Design review of the part built by this model. Coordinates are the model's own, in mm. Face numbers are marked on the shaded views. A direction names the side the tool comes from. Round coordinates to 2 decimals unless told otherwise and drop trailing zeros. Order: outer loops, then holes, each group sorted by start corner. A loop starts at its lowest first (then second) coordinate and runs counter-clockwise, first axis right, second up. Notation, with made-up numbers: (53.5, -28.75) - (85.5, -28.75) arc R4 cw to (85.5, -21.75) - close; hole circle Ø6 at (-2.75, 65.25). An arc over 180 degrees is marked (long way). Use CSV: the item, a comma, the result in double quotes.
Autodesk Inventor part; units mm, degrees
ref_plane "YZ Plane" through (0, 0, 0) normal (1, 0, 0) x (0, 1, 0)
ref_plane "XZ Plane" through (0, 0, 0) normal (0, 1, 0) x (-1, 0, 0)
ref_plane "XY Plane" through (0, 0, 0) normal (0, 0, 1) x (1, 0, 0)
sketch "Sketch1" plane through (0, 0, 0) normal (0, 1, 0) x (-1, 0, 0)
  line L0 (-7.5, 5.5) -> (7.5, 5.5)
  line L1 (7.5, 5.5) -> (7.5, -5.5)
  line L2 (7.5, -5.5) -> (-7.5, -5.5)
  line L3 (-7.5, -5.5) -> (-7.5, 5.5)
  line L4 (-7.5, 5.5) -> (7.5, -5.5) construction
  line L5 (7.5, 5.5) -> (-7.5, -5.5) construction
  circle A0 centre (0, -5.5) radius 7.5 construction
  arc A1 (-7.5, -5.5) -> (7.5, -5.5) centre (0, -5.5) ccw
  point P0 (0, 0)
  dimension "d0" = 11
  dimension "d1" = 15
extrude "Extrusion1" add sketch "Sketch1" along normal blind 8
sketch "Sketch2" plane through (0, 0, 0) normal (0, -1, 0) x (1, 0, 0)
  line L0 (7.5, 9.25) -> (-7.5, 9.25)
  line L1 (-7.5, 9.25) -> (-7.5, -20.75)
  line L2 (-7.5, -20.75) -> (7.5, -20.75)
  line L3 (7.5, -20.75) -> (7.5, 9.25)
  line L4 (7.5, 9.25) -> (-7.5, -20.75) construction
  line L5 (-7.5, 9.25) -> (7.5, -20.75) construction
  line L6 (-7.5, 5.5) -> (7.5, 5.5)
  line L7 (7, 8.75) -> (-7, 8.75) construction
  line L8 (-7, 8.75) -> (-7, -20.25) construction
  line L9 (-7, -20.25) -> (7, -20.25) construction
  line L10 (7, -20.25) -> (7, 8.75) construction
  line L11 (7, 8.75) -> (-7, -20.25) construction
  line L12 (-7, 8.75) -> (7, -20.25) construction
  point P0 (0, 0)
  point P1 (0, -5.75)
  dimension "d4" = 15
  dimension "d5" = 30
  dimension "d6" = 3.75
  dimension "d18" = 0.5
  dimension "d19" = 0.5
sketch "Sketch4" plane through (0, 0, 0) normal (0, -1, 0) x (1, 0, 0)
  line L0 (-7.5, -5.5) -> (-7.5, 5.5)
  line L1 (-7.5, 3.75) -> (-6.5, 3.75)
  line L2 (-6.5, 3.75) -> (-6.5, 0.75)
  line L3 (-6.5, 0.75) -> (-7.5, 0.75)
  line L4 (-7.5, 0.75) -> (-7.5, 3.75)
  line L5 (7.5, 5.5) -> (7.5, -5.5)
  line L6 (7.5, 0.75) -> (6.5, 0.75)
  line L7 (6.5, 0.75) -> (6.5, 3.75)
  line L8 (6.5, 3.75) -> (7.5, 3.75)
  line L9 (7.5, 3.75) -> (7.5, 0.75)
  line L10 (-7.5, -20.25) -> (7.5, -20.25) construction
  line L11 (7.5, -20.25) -> (7.5, 9.75) construction
  line L12 (7.5, 9.75) -> (-7.5, 9.75) construction
  line L13 (-7.5, 9.75) -> (-7.5, -20.25) construction
  line L14 (-7.5, -20.25) -> (7.5, 9.75) construction
  line L15 (7.5, -20.25) -> (-7.5, 9.75) construction
  line L16 (-7.5, 5.5) -> (7.5, 5.5) construction
  arc A0 (-7.5, -5.5) -> (7.5, -5.5) centre (0, -5.5) ccw construction
  point P0 (0, 0)
  point P1 (0, -5.25)
  point P2 (0, -13)
  point P3 (-7, 3.75)
  point P4 (-7.5, 0.75)
  point P5 (-7, 0.75)
  point P6 (7.5, 3.75)
  point P7 (-7.5, 0.75)
  dimension "d20" = 1
  dimension "d21" = 3
  dimension "d22" = 1
  dimension "d23" = 3
  dimension "d24" = 15
  dimension "d25" = 30
  dimension "d27" = 7.25
  dimension "d106" = 0.75
extrude "Extrusion3" add sketch "Sketch4" along normal blind 1.6
sketch "Sketch6" plane through (0, 0, 0) normal (0, -1, 0) x (1, 0, 0)
  line L0 (7.5, 11.25) -> (-7.5, 11.25)
  line L1 (-7.5, 11.25) -> (-7.5, -18.75)
  line L2 (-7.5, -18.75) -> (7.5, -18.75)
  line L3 (7.5, -18.75) -> (7.5, 11.25)
  line L4 (7.5, 11.25) -> (-7.5, -18.75) construction
  line L5 (-7.5, 11.25) -> (7.5, -18.75) construction
  line L6 (7, 10.75) -> (-7, 10.75) construction
  line L7 (-7, 10.75) -> (-7, -18.25) construction
  line L8 (-7, -18.25) -> (7, -18.25) construction
  line L9 (7, -18.25) -> (7, 10.75) construction
  line L10 (7, 10.75) -> (-7, -18.25) construction
  line L11 (-7, 10.75) -> (7, -18.25) construction
  circle A0 centre (0, -3.75) radius 1
  circle A1 centre (0, -3.75) radius 1.5
  line L12 (-6.5, 4.5) -> (6.5, 4.5)
  line L13 (6.5, 4.5) -> (6.5, -5.5)
  line L14 (6.5, -5.5) -> (-6.5, -5.5)
  line L15 (-6.5, -5.5) -> (-6.5, 4.5)
  line L16 (-7.5, 5.5) -> (7.5, 5.5)
  arc A2 (-7.5, -5.5) -> (7.5, -5.5) centre (0, -5.5) ccw
  circle A3 centre (0, -5.5) radius 6.5
  point P0 (0, 0)
  point P1 (-7.5, -3.75)
  point P2 (6.5, -5.5)
  dimension "d31" = 15
  dimension "d32" = 30
  dimension "d34" = 0.5
  dimension "d35" = 0.5
  dimension "d36" = 2
  dimension "d37" = 0.5
  dimension "d38" = 1
  dimension "d39" = 1
  dimension "d40" = 1
  dimension "d41" = 1
  dimension "d107" = 3.75
extrude "Extrusion4" cut sketch "Sketch6" against normal blind 2.5 contours A0 | L12 L13 A3 L15 | A3 L14 | L14 A3
sketch "Sketch10" plane through (0, 8, 0) normal (0, 1, 0) x (1, 0, 0)
  point P0 (0, 0)
sketch "Sketch11" plane through (0, 0, 0) normal (0, -1, 0) x (1, 0, 0)
  line L0 (-5, 3.5) -> (-2.5, 3.5)
  line L1 (-2.5, 3.5) -> (-2.5, 2)
  line L2 (-2.5, 2) -> (-5, 2)
  line L3 (-5, 2) -> (-5, 3.5)
  line L4 (2.5, 3.5) -> (5, 3.5)
  line L5 (5, 3.5) -> (5, 2)
  line L6 (5, 2) -> (2.5, 2)
  line L7 (2.5, 2) -> (2.5, 3.5)
  line L8 (-6.5, 3.75) -> (-7.5, 3.75)
  line L9 (-6.5, 0.75) -> (-6.5, 3.75)
  line L10 (6.5, 3.75) -> (6.5, 0.75)
  line L11 (-6.5, 4.5) -> (6.5, 4.5)
  line L12 (-1.25, -11) -> (1.25, -11)
  line L13 (1.25, -11) -> (1.25, -9.5)
  line L14 (1.25, -9.5) -> (-1.25, -9.5)
  line L15 (-1.25, -9.5) -> (-1.25, -11)
  circle A0 centre (0, -3.75) radius 1
  point P0 (0, 0)
  point P1 (-3.75, 3.5)
  point P2 (3.75, 3.5)
  point P3 (1.25, -10.25)
  point P4 (2.5, 2.75)
  point P5 (0, -9.5)
  point P6 (3.75, 2)
  point P7 (-2.5, 2.75)
  dimension "d51" = 2.5
  dimension "d52" = 1.5
  dimension "d55" = 2.75
  dimension "d56" = 2.75
  dimension "d60" = 13
  dimension "d61" = 3.75
  dimension "d62" = 3.75
  dimension "d103" = 6.5
  dimension "d104" = 6.5
extrude "Extrusion8" cut sketch "Sketch11" against normal blind 10 contours L0 L1 L2 L3 | L4 L5 L6 L7 | L15 L14 L13 L12
sketch "Sketch12" plane through (0, 2.5, 0) normal (0, -1, 0) x (1, 0, 0)
  line L0 (5, 2) -> (5, 3.5) construction
  line L1 (2.5, 2) -> (5, 2) construction
  line L2 (5, 3.5) -> (2.5, 3.5) construction
  line L3 (2.5, 3.5) -> (2.5, 2) construction
  line L4 (2.5, 2) -> (5, 2) construction
  line L5 (5, 2) -> (5, 3.5) construction
  line L6 (-2.5, 2) -> (-2.5, 3.5) construction
  line L7 (-2.5, 2) -> (-5, 2) construction
  line L8 (-2.5, 3.5) -> (-5, 3.5) construction
  line L9 (-5, 3.5) -> (-5, 2) construction
  line L10 (-5, 2) -> (-2.5, 2) construction
  line L11 (-2.5, 2) -> (-2.5, 3.5) construction
  line L12 (-1.25, -9.5) -> (1.25, -9.5) construction
  line L13 (-1.25, -9.5) -> (-1.25, -11) construction
  line L14 (1.25, -9.5) -> (-1.25, -9.5) construction
  line L15 (-1.25, -9.5) -> (-1.25, -11) construction
  line L16 (-1.25, -11) -> (1.25, -11) construction
  line L17 (1.25, -11) -> (1.25, -9.5) construction
  line L18 (5.5, 3.5) -> (2, 3.5)
  line L19 (2, 3.5) -> (2, 2)
  line L20 (2, 2) -> (5.5, 2)
  line L21 (5.5, 2) -> (5.5, 3.5)
  line L22 (1.75, -9.5) -> (-1.75, -9.5)
  line L23 (-1.75, -9.5) -> (-1.75, -11)
  line L24 (-1.75, -11) -> (1.75, -11)
  line L25 (1.75, -11) -> (1.75, -9.5)
  line L26 (-2, 3.5) -> (-5.5, 3.5)
  line L27 (-5.5, 3.5) -> (-5.5, 2)
  line L28 (-5.5, 2) -> (-2, 2)
  line L29 (-2, 2) -> (-2, 3.5)
  point P0 (0, 0)
  point P1 (-2.5, 2.75)
  point P2 (-2, 2.75)
  point P3 (-3.75, 2)
  point P4 (-3.75, 2)
  point P5 (-3.75, 3.5)
  point P6 (-3.75, 3.5)
  point P7 (-5, 2.75)
  point P8 (-5.5, 2.75)
  point P9 (1.25, -10.25)
  point P10 (1.75, -10.25)
  point P11 (0, -11)
  point P12 (-1.25, -10.25)
  dimension "d63" = 0.5
  dimension "d64" = 0
  dimension "d65" = 0
  dimension "d67" = 0.5
  dimension "d68" = 0
  dimension "d69" = 0
  dimension "d70" = 0.5
  dimension "d71" = 0.5
  dimension "d72" = 0
  dimension "d73" = 0
  dimension "d74" = 0.5
  dimension "d96" = 0.5
extrude "Extrusion9" cut sketch "Sketch12" against normal blind 1
sketch "Sketch16" plane through (0, 2.5, 0) normal (0, -1, 0) x (1, 0, 0)
  line L0 (-6.5, -5.5) -> (-6.5, 4.5) construction
  line L1 (-6.5, 4.5) -> (6.5, 4.5) construction
  line L2 (-6.5, 4.5) -> (6.5, 4.5) construction
  line L3 (-0.5, 4.5) -> (0.5, 4.5)
  line L4 (0.5, 4.5) -> (0.5, -2.75)
  line L5 (0.5, -2.75) -> (-0.5, -2.75)
  line L6 (-0.5, -2.75) -> (-0.5, 4.5)
  circle A0 centre (0, -3.75) radius 1.5 construction
  circle A1 centre (0, -3.75) radius 1.75 construction
  line L7 (-6.5, -2.75) -> (6.5174, -2.75) construction
  circle A2 centre (0, -3.75) radius 1.5 construction
  circle A3 centre (0, -3.75) radius 1 construction
  line L8 (6.5, 0.75) -> (6.5, -5.5)
  line L9 (-6.5, -5.873) -> (6.5, -5.873)
  line L10 (6.5, -5.873) -> (6.5, -6.873)
  line L11 (6.5, -6.873) -> (-6.5, -6.873)
  line L12 (-6.5, -6.873) -> (-6.5, -5.873)
  point P0 (0, 0)
  point P1 (0, 4.5)
  point P2 (0.0087, -2.75)
  dimension "d94" = 1
  dimension "d95" = 1
extrude "Extrusion10" add sketch "Sketch16" along normal blind 2.5 contours L3 L4 L5 L6
sketch "Sketch19" plane through (-7.5, 0, 5.5) normal (0, 0, 1) x (1, 0, 0)
  line L0 (15, 0) -> (15, 8)
  line L1 (0, 8) -> (15, 8)
  line L2 (15, 8) -> (15, 0)
  line L3 (15, 0) -> (0, 0)
  line L4 (0, 0) -> (0, 8)
  point P0 (7.5, 0)
extrude "Extrusion13" add sketch "Sketch19" along normal blind 6
sketch "Sketch18" plane through (0, 8, 0) normal (0, 1, 0) x (1, 0, 0)
  line L0 (-7.5, -3.75) -> (-7.5, -5.5)
  line L1 (-7.5, -5.5) -> (-7.5, -8.2917)
  line L2 (7.5, -5.5) -> (7.5, -8.2917)
  arc A0 (7.5, -8.2917) -> (-7.5, -8.2917) centre (0, -17.6592) ccw
  line L3 (-7.5, -5.5) -> (0, -3.75)
  line L4 (-7.5, -5.5) -> (7.5, -5.5)
  line L5 (0, -3.75) -> (7.5, -5.5)
  line L6 (-7.5, -8.2917) -> (-7.5, -17.8663)
  line L7 (-7.5, -17.8663) -> (8.2387, -17.8663)
  line L8 (8.2387, -17.8663) -> (7.5, -8.2917)
  line L9 (-7.5, -8.2917) -> (-7.5, -5.5)
  point P0 (0, 0)
  point P1 (3.395, -5.5)
  point P2 (-3.395, -5.5)
  dimension "d108" = 12
extrude "Extrusion12" cut sketch "Sketch18" against normal blind 8 contours A0 L8 L7 L6
sketch "Sketch21" plane through (0, 8, 0) normal (0, 1, 0) x (1, 0, 0)
  line L0 (-7.5, 5.5) -> (-7.5, -8.2917)
  line L1 (-7.5, 5.5) -> (-4.5586, 5.5)
  line L2 (-4.5586, 5.5) -> (-4.5586, 13.4633)
  line L3 (-4.5586, 13.4633) -> (-7.5, 13.4633)
  line L4 (-7.5, 13.4633) -> (-7.5, 5.5)
  arc A0 (7.5, 5.5) -> (-7.5, 5.5) centre (0, 5.5) ccw
  line L5 (7.5, 5.5) -> (3.8632, 5.5)
  line L6 (3.8632, 5.5) -> (3.8632, 13.1156)
  line L7 (3.8632, 13.1156) -> (7.5, 13.1156)
  line L8 (7.5, 13.1156) -> (7.5, 5.5)
  point P0 (0, 0)
  point P1 (3.8632, 11.9285)
  point P2 (-4.5586, 11.4556)
  point P3 (-7.5, -5.5)
extrude "Extrusion15" add sketch "Sketch21" against normal blind 8 contours L6 L7 L8 A0 | L4 L3 L2 A0
sketch "Sketch20" plane through (0, 8, 0) normal (0, 1, 0) x (1, 0, 0)
  arc A0 (7.5, 5.5) -> (-7.5, 5.5) centre (0, 5.5) ccw
  line L0 (-7.5, 5.5) -> (-7.5, 7.5)
  line L1 (7.5, 5.5) -> (7.5, 7.5)
  arc A1 (0, 13) -> (-7.5, 7.5) centre (1.4853, 3.1109) ccw
  arc A2 (7.5, 7.5) -> (0, 13) centre (-1.4853, 3.1109) ccw
  line L2 (-7.5, 7.5) -> (-7.5, 19.3065)
  line L3 (-7.5, 7.5) -> (4.3065, 7.5) construction
  line L4 (-7.5, 19.3065) -> (7.5, 19.3065)
  line L5 (7.5, 19.3065) -> (7.5, 7.5)
  point P0 (0, 0)
  point P1 (-6.7259, 8.8184)
  point P2 (6.7259, 8.8184)
  dimension "d113" = 2
  dimension "d114" = 10
  dimension "d115" = 90
  dimension "d116" = 90
extrude "Extrusion14" cut sketch "Sketch20" against normal blind 10 contours A2 A0 | A0 A1 L2 L4 L5 A2 | A1 A0
sketch "Sketch23" plane through (0, 2.5, -3.75) normal (0, -1, 0) x (1, 0, 0)
  circle A0 centre (0, 0) radius 1
  circle A1 centre (0, 0) radius 1
  point P0 (0, 3.75)
extrude "Extrusion17" cut sketch "Sketch23" against normal blind 4
sketch "Sketch22" plane through (0, 8, 0) normal (0, 1, 0) x (1, 0, 0)
  line L0 (7.5, 7.5) -> (7.5, -8.2917)
  line L1 (-7.5, 7.5) -> (-7.5, -8.2917)
  arc A0 (7.5, -7.2917) -> (-7.5, -7.2917) centre (0, -16.6592) ccw
  line L2 (-7.5, -7.2917) -> (7.5, -7.2917) construction
  line L3 (-7.5, -7.2917) -> (7.5, -7.2917) construction
  arc A1 (7.5, -8.2917) -> (-7.5, -8.2917) centre (0, -17.6592) ccw
  arc A2 (7.5, -6.2917) -> (-7.5, -6.2917) centre (0, -15.6592) ccw
  line L4 (-7.5, -6.2917) -> (7.5, -6.2917) construction
  line L5 (-7.5, -6.2917) -> (7.5, -6.2917) construction
  point P0 (0, 0)
  point P1 (0, -4.6592)
  point P2 (0, -5.6592)
  point P3 (0, -3.6592)
  dimension "d121" = 0
  dimension "d122" = 1
  dimension "d123" = 1
  dimension "d124" = 0
  dimension "d125" = 1
  dimension "d126" = 1
sketch "Sketch14" plane through (0, 2.5, 0) normal (0, -1, 0) x (1, 0, 0)
  line L0 (5, 2.75) -> (2.5, 2.75) construction
  line L1 (2.5, 2.75) -> (2.5, 1.25) construction
  line L2 (2.5, 1.25) -> (5, 1.25) construction
  line L3 (5, 1.25) -> (5, 2.75) construction
  line L4 (5.5, 3.25) -> (2, 3.25)
  line L5 (2, 3.25) -> (2, 0.75)
  line L6 (2, 0.75) -> (5.5, 0.75)
  line L7 (5.5, 0.75) -> (5.5, 3.25)
  dimension "d86" = 0.5
  dimension "d87" = 0.5
sketch "Sketch15" plane through (0, 3.5, 0) normal (0, -1, 0) x (1, 0, 0)
  line L0 (5, 2.75) -> (2.5, 2.75)
  line L1 (2.5, 2.75) -> (2.5, 1.25)
  line L2 (2.5, 1.25) -> (5, 1.25)
  line L3 (5, 1.25) -> (5, 2.75)
  point P0 (0, 0)
sketch "Sketch8" plane through (0, 0, -3.75) normal (0, -1, 0) x (1, 0, 0)
  circle A0 centre (0, 0) radius 1.75
  circle A1 centre (0, 0) radius 1.5
  circle A2 centre (0, 0) radius 1.5
  point P0 (0, 3.75)
  dimension "d46" = 0.25
sketch "Sketch7" plane through (0, 2.5, -3.75) normal (0, -1, 0) x (1, 0, 0)
  circle A0 centre (0, 0) radius 1.25
  point P0 (0, 3.75)
properties part number "ORGATE"
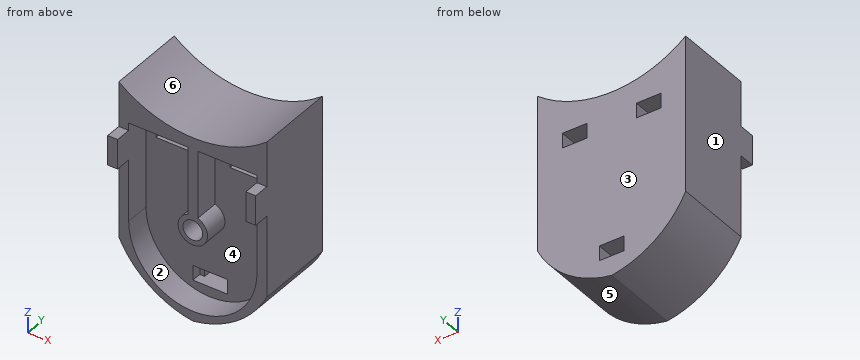
1) Insertion check: pin 1 Ø0.6 at (x, z) = (2.5, 2.5) entering from -Y; pin 2 Ø1 at (x, y) = (4.5, 5) entering from -Z; pin 3 Ø0.6 at (x, z) = (-1.5, -10) entering from -Y. Each pin has a flat end and moves straight along its axis. Give the tip position at first contact, or say it passes through.
Data:
pin 1,"stops at y = 3.5"
pin 2,"stops at z = -11.47"
pin 3,"stops at y = 2.5"
2) We need section A-A (y = 7). Give the boundary of the cut face in (x, z).
Data:
outline,"(-7.5, -7.5) arc R10 ccw to (0, -13) arc R10 ccw to (7.5, -7.5) - (7.5, 8.29) arc R12 cw to (-7.5, 8.29) - close; hole (-5, 2) - (-2.5, 2) - (-2.5, 3.5) - (-5, 3.5) - close; hole (-1.25, -11) - (1.25, -11) - (1.25, -9.5) - (-1.25, -9.5) - close; hole (2.5, 2) - (5, 2) - (5, 3.5) - (2.5, 3.5) - close"
3) The part is to be moulded in two halves that separate along Z. For the marked faces 3, 4, 5 and 6, say which applies: +Z half, -Z half, draft (parallel to the pull), parting line (faces both ways), or undercut.
Data:
face 3,"draft"
face 4,"undercut"
face 5,"-Z half"
face 6,"+Z half"
4) We need section B-B (y = 1). Give the boundary of the cut face in (x, z), then the cut area to 3 significant figures.
Data:
outline,"(-7.5, -7.5) arc R10 ccw to (0, -13) arc R10 ccw to (7.5, -7.5) - (7.5, 8.29) arc R12 cw to (-7.5, 8.29) - close; hole (-6.5, -5.5) arc R6.5 ccw to (6.5, -5.5) - (6.5, 4.5) - (0.5, 4.5) - (0.5, -2.34) arc R1.5 cw (long way) to (-0.5, -2.34) - (-0.5, 4.5) - (-6.5, 4.5) - close; hole circle Ø2 at (0, -3.75)"
area,"79.9 mm2"
5) For the marked faces 1 and 2, list the 3-axis set-ups (+Z, -Z, +X, -X, +Y, -Y) from which the entire face can be reached by the end or side of a thin tool; tool diameter is ignored.
Data:
face 1,"+Z, -Z, -X, +Y, -Y"
face 2,"-Y"
6) We need section C-C (y = 6). Give the boundary of the cut face in (x, z).
Data:
outline,"(-7.5, -7.5) arc R10 ccw to (0, -13) arc R10 ccw to (7.5, -7.5) - (7.5, 8.29) arc R12 cw to (-7.5, 8.29) - close; hole (-5, 2) - (-2.5, 2) - (-2.5, 3.5) - (-5, 3.5) - close; hole (-1.25, -11) - (1.25, -11) - (1.25, -9.5) - (-1.25, -9.5) - close; hole circle Ø2 at (0, -3.75); hole (2.5, 2) - (5, 2) - (5, 3.5) - (2.5, 3.5) - close"
7) We need section D-D (z = -1.25). Give the boundary of the cut face in (x, y), then the cut area to 3 significant figures.
Data:
outline,"(-7.5, 0) - (-6.5, 0) - (-6.5, 2.5) - (-0.5, 2.5) - (-0.5, 0) - (0.5, 0) - (0.5, 2.5) - (6.5, 2.5) - (6.5, 0) - (7.5, 0) - (7.5, 8) - (-7.5, 8) - close"
area,"90.0 mm2"
